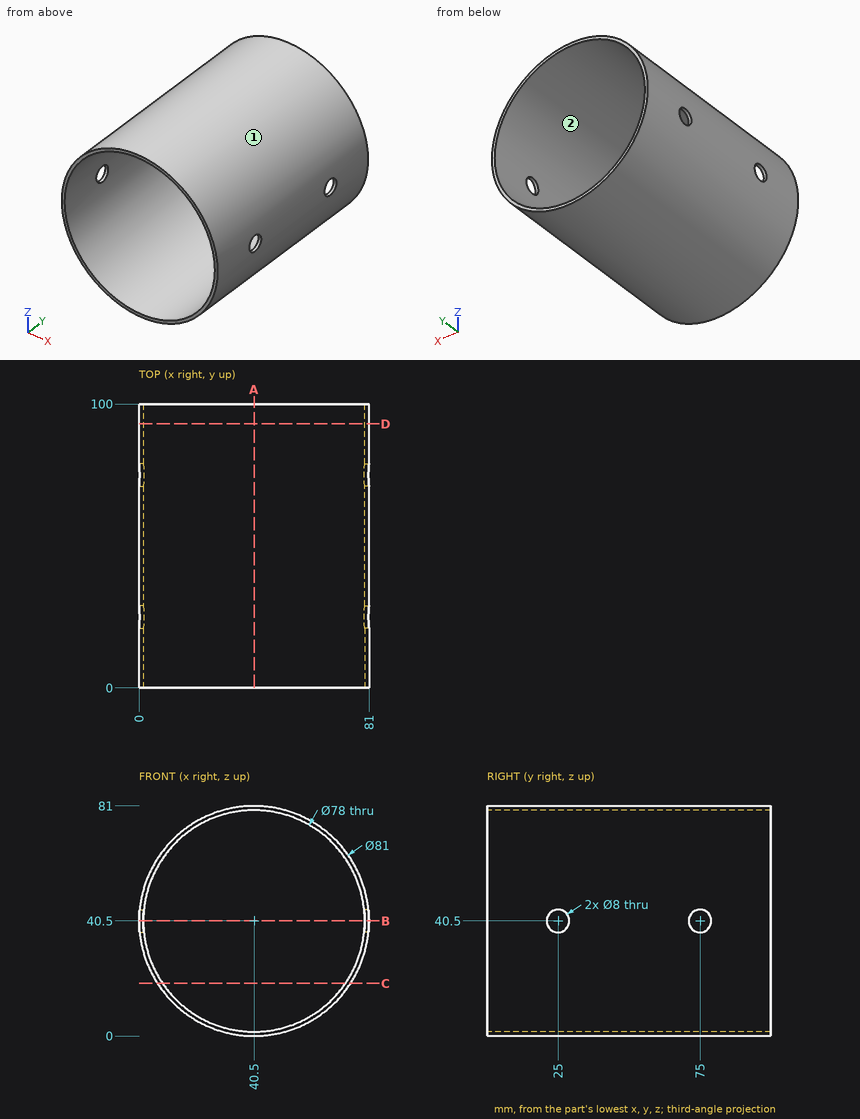
Design review of the part shown in the three views and the two pictorial views. Dimensions are in mm from the part's minimum x, y and z. Coordinates: 2 decimals unless noted, no trailing zeros. Order: outer loops, then holes, each group sorted by start corner. A loop starts at its lowest first (then second) coordinate and runs counter-clockwise, first axis right, second up. Notation, with made-up numbers: (-20, 45.5) - (11, 45.5) arc R33 ccw to (11, 80.5) - close; hole circle Ø11 at (-28, 68.25). An arc over 180 degrees is marked (long way). Answer as CSV lines item,"result". Start each with the question number.
1) Add section B-B (z = 40.5). State the section outline as (x, y) points.
2) Add section C-C (z = 18.5). State the section outline as (x, y) points.
3) Add section D-D (y = 93). State the section outline as (x, z) points, then the cut area to 3 significant figures.
4) Add section A-A (x = 40.5). State the section outline as (y, z) points, then the cut area to 3 significant figures.
5) Insertion check: P1, Ø12, axis at y = 11.5, z = 50, coming from the +X side; P2, Ø5, axis at y = 34.5, z = 57.5, coming from the -X side; P3, Ø7, axis at y = 75, z = 40.5, coming from the +X side; P4, Ø1.5, axis at x = 25, y = 62, coming from the +Z side. Each pin has a flat end and moves straight along its axis. Give the tip position at first contact, or say it passes through.
6) Draft analysis for pull direction Z (two halves, no side actions). For the marked faces 1 and 2, state which applies: +Z half, -Z half, draft (parallel to the pull), parting line (faces both ways), or undercut.
7) To check wall thickness, follow line 1 along X through (y, z) = (20, 40); line 2 along Y through (x, z) = (1, 40). State the ranges of each line that lie inside material, in increasing order. Write a range as [from, to].
Result:
1,outline,"(0, 0) - (1.5, 0) - (1.5, 21) - (0, 21) - close; (0, 29) - (1.5, 29) - (1.5, 71) - (0, 71) - close; (0, 79) - (1.5, 79) - (1.5, 100) - (0, 100) - close; (79.5, 0) - (81, 0) - (81, 21) - (79.5, 21) - close; (79.5, 29) - (81, 29) - (81, 71) - (79.5, 71) - close; (79.5, 79) - (81, 79) - (81, 100) - (79.5, 100) - close"
2,outline,"(6.5, 0) - (8.3, 0) - (8.3, 100) - (6.5, 100) - close; (72.7, 0) - (74.5, 0) - (74.5, 100) - (72.7, 100) - close"
3,outline,"circle Ø81 at (40.5, 40.5); hole circle Ø78 at (40.5, 40.5)"
3,area,"375 mm^2"
4,outline,"(0, 0) - (100, 0) - (100, 1.5) - (0, 1.5) - close; (0, 79.5) - (100, 79.5) - (100, 81) - (0, 81) - close"
4,area,"300 mm^2"
5,P1,"x = 80.85"
5,P2,"x = 2.68"
5,P3,"through"
5,P4,"z = 78.22"
6,face 1,"parting line"
6,face 2,"undercut"
7,line 1,"[0, 1.5], [79.5, 81]"
7,line 2,"[0, 21.03], [28.97, 71.03], [78.97, 100]"
